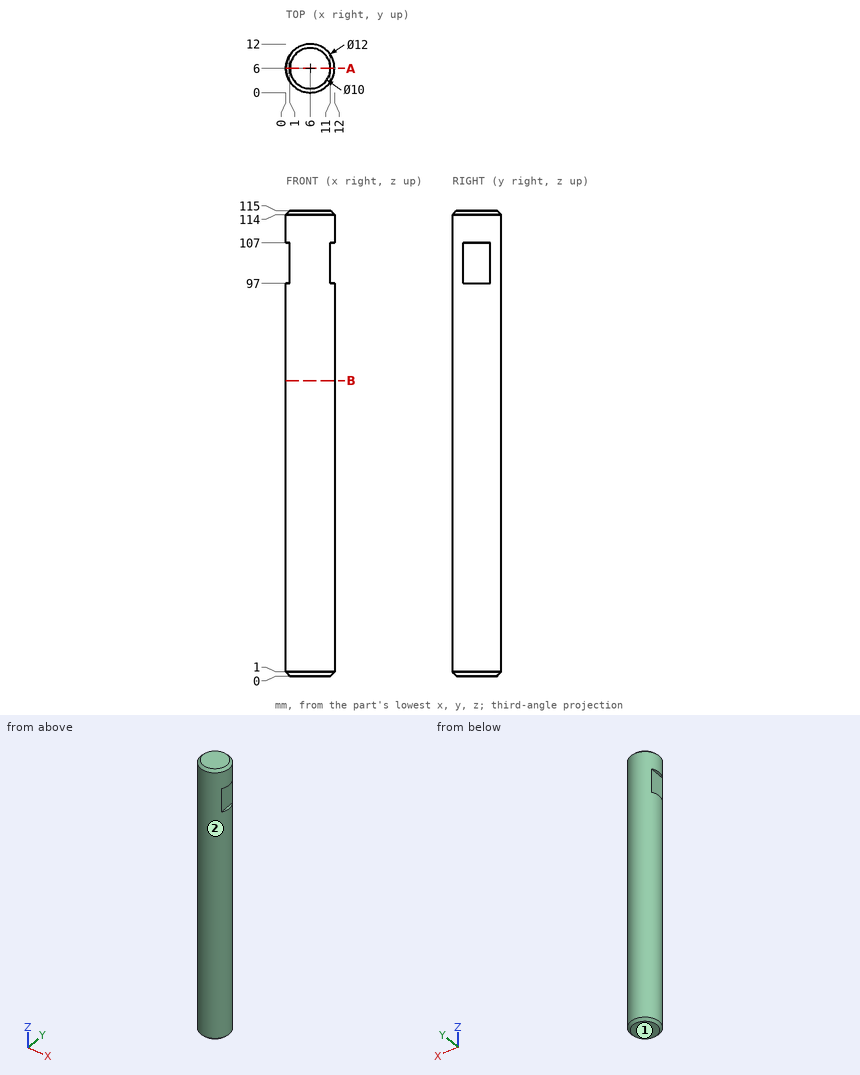
The figure shows three views and two pictorial views of one solid part (mm, origin at its lowest corner). Answer the questions. Round coordinates to 2 decimals unless told otherwise and drop trailing zeros. Order: outer loops, then holes, each group sorted by start corner. A loop starts at its lowest first (then second) coordinate and runs counter-clockwise, first axis right, second up.
Q1. Given pin 1 Ø2 at (x, z) = (3, 90) entering from -Y; pin 2 Ø2 at (y, z) = (5, 101.5) entering from +X; pin 3 Ø0.5 at (x, y) = (11.5, 6) entering from +Z, each flat-ended and moving along its own axis, determine where each tip first touches the part or whether it passes through.
Solution:
pin 1: stops at y = 0.34
pin 2: stops at x = 11
pin 3: stops at z = 114.75
Q2. The mould has two halves that part along X. Classify the marked faces 1 and 2: pulls with the +X half, pulls with the -X half, needs draft (parallel to the pull), parting line crosses it, or undercut.
Solution:
face 1: needs draft
face 2: parting line crosses it
Q3. A cutting plane is placed at A-A, the plane y = 6. Determine the outline of the cut face in (x, z), then the cut area to 3 significant figures.
Solution:
outline: (0, 1) - (1, 0) - (11, 0) - (12, 1) - (12, 97) - (11, 97) - (11, 107) - (12, 107) - (12, 114) - (11, 115) - (1, 115) - (0, 114) - (0, 107) - (1, 107) - (1, 97) - (0, 97) - close
area: 1,360 mm2
Q4. Find the intervals of material crossed by line 1 along Y through (x, z) = (1, 34); line 2 along Y through (x, z) = (6.5, 11); line 3 along X through (y, z) = (0.5, 44), in increasing order.
Solution:
line 1: y = 2.68 to 9.32
line 2: y = 0.02 to 11.98
line 3: x = 3.6 to 8.4
Q5. A cutting plane is placed at B-B, the plane z = 73. Determine the outline of the cut face in (x, y), then the cut area to 3 significant figures.
Solution:
outline: circle Ø12 at (6, 6)
area: 113 mm2
